Geometry: see drawing. Coordinates: mm, zero at the bounding-box minimum. A direction names the side the tool comes from. Coordinates: 2 decimals unless noted, no trailing zeros. Order: outer loops, then holes, each group sorted by start corner. A loop starts at its lowest first (then second) coordinate and runs counter-clockwise, first axis right, second up.
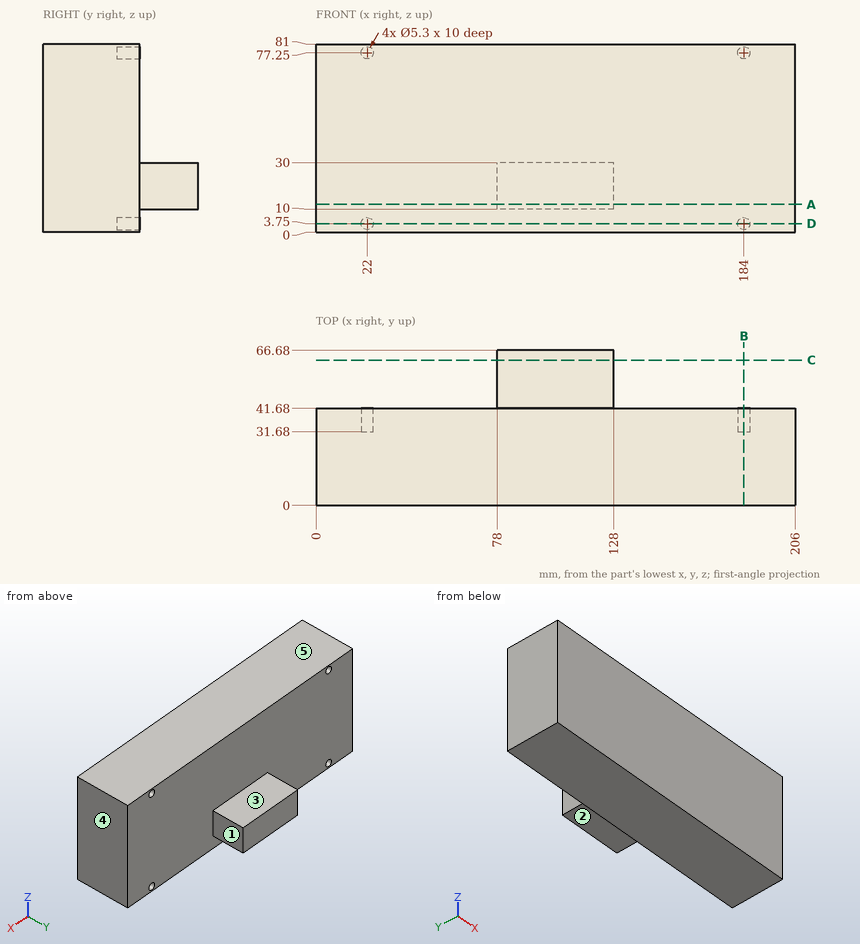
Q1. Section query C-C on y = 62.5. Output: boundary loops of the cut face in (x, z), plus the area to 3 significant figures.
Solutions:
outline: (78, 10) - (128, 10) - (128, 30) - (78, 30) - close
area: 1,000 mm2
Q2. Section query A-A on z = 12. Output: boundary loops of the cut face in (x, y), plus the area to 3 significant figures.
Solutions:
outline: (0, 0) - (206, 0) - (206, 41.68) - (128, 41.68) - (128, 66.68) - (78, 66.68) - (78, 41.68) - (0, 41.68) - close
area: 9,840 mm2
Q3. Set-up query: the marked faces 1, 2, 3, 4 and 5. Return all of +Z, -Z, +X, -X, +Y, -Y with unobstructed straight access to the full face (end or side cutting, diameter ignored); none if empty.
Solutions:
face 1: +Z, -Z, +X, +Y
face 2: -Z, +X, -X, +Y
face 3: +Z, +X, -X, +Y
face 4: +Z, -Z, +X, +Y, -Y
face 5: +Z, +X, -X, +Y, -Y
Q4. Section query B-B on x = 184. Output: boundary loops of the cut face in (y, z).
Solutions:
outline: (0, 0) - (41.68, 0) - (41.68, 1.1) - (31.68, 1.1) - (31.68, 6.4) - (41.68, 6.4) - (41.68, 74.6) - (31.68, 74.6) - (31.68, 79.9) - (41.68, 79.9) - (41.68, 81) - (0, 81) - close
Q5. Material intervals for line 1 along Z through (x, y) = (184, 39); line 2 along X through (y, z) = (35.25, 77.25); line 3 along X through (y, z) = (33, 75.5), sorted ascending.
Solutions:
line 1: z = 0 to 1.1, 6.4 to 74.6, 79.9 to 81
line 2: x = 0 to 19.35, 24.65 to 181.35, 186.65 to 206
line 3: x = 0 to 20.01, 23.99 to 182.01, 185.99 to 206
Q6. Pin query (flat end, axial travel): P1, Ø6, axis at x = 21.5, z = 4.5, coming from the +Y side; P2, Ø20, axis at x = 107, y = 57.5, coming from the +Z side; P3, Ø22, axis at y = 55.5, z = 18.5, coming from the -X side. Return the tip coordinate at first contact, or that it passes through.
Solutions:
P1: stops at y = 41.68
P2: stops at z = 30
P3: stops at x = 78
Q7. Section query D-D on z = 3.75. Output: boundary loops of the cut face in (x, y).
Solutions:
outline: (0, 0) - (206, 0) - (206, 41.68) - (186.65, 41.68) - (186.65, 31.68) - (181.35, 31.68) - (181.35, 41.68) - (24.65, 41.68) - (24.65, 31.68) - (19.35, 31.68) - (19.35, 41.68) - (0, 41.68) - close
